For this review, take the finished solid that the model builds, in its own axes (mm). Face numbers are marked on the shaded views. A direction names the side the tool comes from. Round coordinates to 2 decimals unless told otherwise and drop trailing zeros. Write each loop counter-clockwise with the first axis right and the second up, starting at its lowest first coordinate (ties: lowest second). Pieces come first, ordered by that corner, then holes. Notation, with made-up numbers: M 13,-7.5 L 53,-7.5 A30 ccw 53,23.5 Z; hole C -27.75,-37.5 d6. An arc over 180 degrees is marked long. Use one line per item in the form item = value. Start each with the question number.
Item 1: Draft analysis for pull direction X (two halves, no side actions). For the marked faces 1 and 2, state which applies: released by +X, released by -X, zero draft, split by the parting line, or undercut.
Item 2: For line 1 (Y direction, x = 0, z = -12); line 2 (Z direction, x = -6, y = -10); line 3 (Y direction, x = 4, z = -23), list the stretches that pass through material, from the lowest coordinate up. Write a range as [from, to].
Item 3: For P1, Ø5, axis at x = -16.5, z = 8.5, coming from the +Y side; P2, Ø3, axis at x = 30, y = -10, coming from the +Z side; P3, Ø3, axis at y = 20.5, z = 21, coming from the +X side; P4, Ø11, axis at x = 0, y = 0, coming from the +Z side, all flat-tipped, find the tip position at first contact; note any pin that passes through.
Item 4: For the marked faces 3 and 4, list the 3-axis set-ups (+Z, -Z, +X, -X, +Y, -Y) from which the entire face can be reached by the end or side of a thin tool; tool diameter is ignored.
Item 5: Add section A-A (y = 0). State the section outline as (x, z) points, and give its area (3 significant figures).
Item 6: Add section C-C (z = -4). State the section outline as (x, y) points, and give its area (3 significant figures).
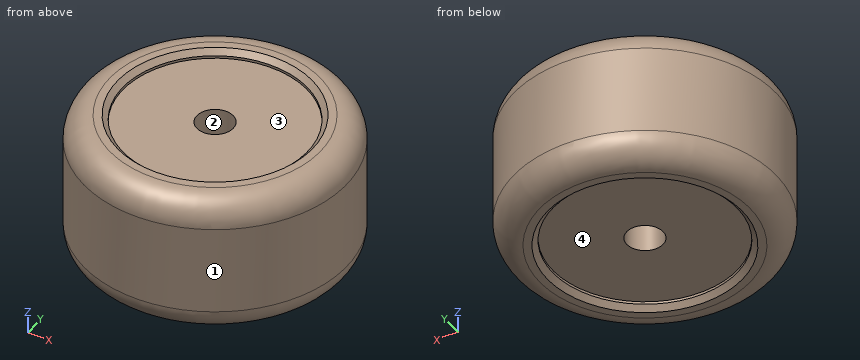
Autodesk Inventor part; units mm, degrees
ref_plane "YZ Plane" through (0, 0, 0) normal (1, 0, 0) x (0, 1, 0)
ref_plane "XZ Plane" through (0, 0, 0) normal (0, 1, 0) x (-1, 0, 0)
ref_plane "XY Plane" through (0, 0, 0) normal (0, 0, 1) x (1, 0, 0)
sketch "Sketch2" plane through (0, 0, 0) normal (0, 0, 1) x (1, 0, 0)
  circle A0 centre (0, 0) radius 50.5
  circle A1 centre (0, 0) radius 47.5
  circle A2 centre (0, 0) radius 35.5
  circle A3 centre (0, 0) radius 7
  dimension "d0" = 101
  dimension "d1" = 3
  dimension "d2" = 15
  dimension "d3" = 14
extrude "Extrusion1" add sketch "Sketch2" along normal blind 27 and the other way blind 27 contours A0 | A1 | A2
extrude "Extrusion2" cut sketch "Sketch2" against normal blind 3 from surface at 27 contours A2
extrude "Extrusion3" cut sketch "Sketch2" along normal blind 3 from surface at -27 contours A2
chamfer "Chamfer1" distance 2 angle 45 2 edges at (-35.5, 0, 27) (-35.5, 0, -27)
fillet "Fillet1" radius 10 2 edges at (-50.5, 0, -27) (-50.5, 0, 27)
properties part number "wheel_stand_in"
Calculated:
q1.face_1 = split by the parting line
q1.face_2 = undercut
q2.line_1 = [-50.5, -7], [7, 50.5]
q2.line_2 = [-24, 24]
q2.line_3 = [-48.33, -5.74], [5.74, 48.33]
q3.P1 = 48.52
q3.P2 = 24
q3.P3 = 46.13
q3.P4 = through
q4.face_3 = +Z
q4.face_4 = -Z
q5.outline = M -50.5,-17 A10 ccw -40.5,-27 L -37.5,-27 L -35.5,-25 L -35.5,-24 L -7,-24 L -7,24 L -35.5,24 L -35.5,25 L -37.5,27 L -40.5,27 A10 ccw -50.5,17 Z; M 7,-24 L 35.5,-24 L 35.5,-25 L 37.5,-27 L 40.5,-27 A10 ccw 50.5,-17 L 50.5,17 A10 ccw 40.5,27 L 37.5,27 L 35.5,25 L 35.5,24 L 7,24 Z
q5.area = 4,260 mm^2
q6.outline = C 0,0 d101; hole C 0,0 d14
q6.area = 7,860 mm^2
